Part model, mm, in its own coordinate system. Face numbers are marked on the shaded views. A direction names the side the tool comes from. Round coordinates to 2 decimals unless told otherwise and drop trailing zeros. Order: outer loops, then holes, each group sorted by start corner. A loop starts at its lowest first (then second) coordinate and runs counter-clockwise, first axis right, second up. Notation, with made-up numbers: (43, 4.25) - (95, 4.25) arc R20 cw to (95, 43.25) - close; hole circle Ø2 at (0.5, -38.75). An arc over 180 degrees is marked (long way). Return JSON: item names as keys, results as strings. Group by question number.
Item 1: Two-plate mould, pull along Y, no slides. Class the marked faces 3, 4, 5 and 6: released by +Y, released by -Y, zero draft, split by the parting line, or undercut.
Item 2: Tool access for the marked faces 1 and 2: list every direction of +Z, -Z, +X, -X, +Y, -Y with a clear straight run to the whole face (end or side of a thin tool).
Item 3: Saw through at D-D on x = 0. List the corners of the cut face in (y, z), and give its area (3 significant figures).
Item 4: Drop a flat-ended pin along its axis: pin 1 (1.5 mm diameter, centred on x = 1.5, z = -0.5, fed in from -Y). Give the stop position or say it passes through.
Item 5: Saw through at C-C on z = 0. List the corners of the cut face in (x, y), and give its area (3 significant figures).
Item 6: Saw through at B-B on z = -1.55. List the corners of the cut face in (x, y).
Item 7: Saw through at A-A on x = 2. List the corners of the cut face in (y, z).
Item 8: Probe probe 1 along Y at (x, z) = (1.15, -2.25); probe 2 along Z at (x, y) = (0, 3.95); probe 3 along Z at (x, y) = (-0.6, 3.4). List the from-to ranges inside material, lowest first.
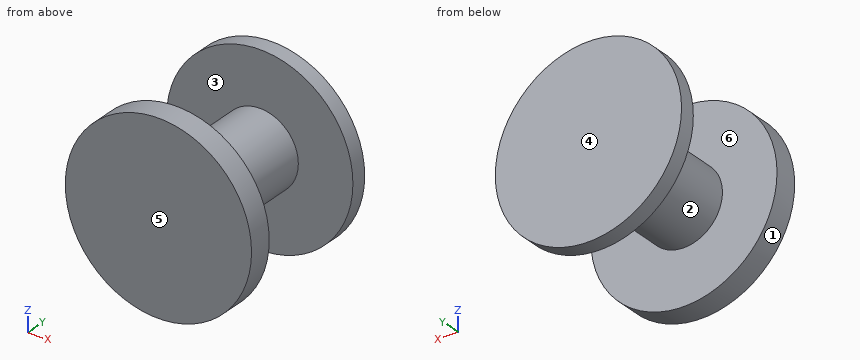
```python
from build123d import *

# Parameters (mm, degrees)
SKETCH1_R           = 2.9
BOSS_EXTRUDE1_DEPTH = 0.75
SKETCH2_R           = 1.2
BOSS_EXTRUDE2_DEPTH = 3.55
SKETCH3_R           = 2.9
BOSS_EXTRUDE3_DEPTH = 0.5


with BuildPart() as part:
    # Sketch1 → Boss-Extrude1 (new body)
    with BuildSketch(Plane(origin=(0, 0, 0), x_dir=(1, 0, 0), z_dir=(0, 1, 0))):
        Circle(SKETCH1_R)
    extrude(amount=BOSS_EXTRUDE1_DEPTH)

    # Sketch2 → Boss-Extrude2 (add)
    with BuildSketch(Plane(origin=(0, 0.75, 0), x_dir=(1, 0, 0), z_dir=(0, 1, 0))):
        Circle(SKETCH2_R)
    extrude(amount=BOSS_EXTRUDE2_DEPTH)

    # Sketch3 → Boss-Extrude3 (add)
    with BuildSketch(Plane(origin=(0, 4.3, 0), x_dir=(1, 0, 0), z_dir=(0, 1, 0))):
        Circle(SKETCH3_R)
    extrude(amount=BOSS_EXTRUDE3_DEPTH)


solid = part.part
```
Filled in:
{
 "1": {"face 3": "undercut", "face 4": "released by +Y", "face 5": "released by -Y", "face 6": "undercut"},
 "2": {"face 1": "+Y, -Y", "face 2": "none"},
 "3": {"outline": "(0, -2.9) - (0.75, -2.9) - (0.75, -1.2) - (4.3, -1.2) - (4.3, -2.9) - (4.8, -2.9) - (4.8, 2.9) - (4.3, 2.9) - (4.3, 1.2) - (0.75, 1.2) - (0.75, 2.9) - (0, 2.9) - close", "area": "15.8 mm^2"},
 "4": {"pin 1": "stops at y = 0"},
 "5": {"outline": "(-2.9, 0) - (2.9, 0) - (2.9, 0.75) - (1.2, 0.75) - (1.2, 4.3) - (2.9, 4.3) - (2.9, 4.8) - (-2.9, 4.8) - (-2.9, 4.3) - (-1.2, 4.3) - (-1.2, 0.75) - (-2.9, 0.75) - close", "area": "15.8 mm^2"},
 "6": {"outline": "(-2.45, 0) - (2.45, 0) - (2.45, 0.75) - (-2.45, 0.75) - close; (-2.45, 4.3) - (2.45, 4.3) - (2.45, 4.8) - (-2.45, 4.8) - close"},
 "7": {"outline": "(0, -2.1) - (0.75, -2.1) - (0.75, 2.1) - (0, 2.1) - close; (4.3, -2.1) - (4.8, -2.1) - (4.8, 2.1) - (4.3, 2.1) - close"},
 "8": {"probe 1": "y = 0 to 0.75, 4.3 to 4.8", "probe 2": "z = -1.2 to 1.2", "probe 3": "z = -1.04 to 1.04"}
}
